Could you check a few things on this model? Use its own coordinates, in mm. Face numbers are marked on the shaded views. A direction names the side the tool comes from. Round coordinates to 2 decimals unless told otherwise and drop trailing zeros. Order: outer loops, then holes, each group sorted by start corner. A loop starts at its lowest first (then second) coordinate and runs counter-clockwise, first axis right, second up. Notation, with made-up numbers: M 26,84.25 L 40,84.25 A20 cw 40,110.25 Z; hole C 60,-14 d7. An arc over 180 degrees is marked long. Write each question's results on one line, items separated by ' | '. Start each with the question number.
1. Suppose I cut it at A-A on y = 176. Write out the boundary of the cut face in (x, z).
2. We'd pull the mould along X, two halves only. Please class the marked faces 1, 2 and 3: released by +X, released by -X, zero draft, split by the parting line, or undercut.
3. Suppose I cut it at B-B on x = 201. Write out the boundary of the cut face in (y, z), and give its area (3 significant figures).
4. I'm going to push a flat-ended pin straight in: pin 1 (1 mm diameter, centred on x = 204.5, y = 175.5, fed in from -Z). Where does the tip first touch, or does it pass through?
5. For the marked faces 4 and 5, which set-ups out of +Z, -Z, +X, -X, +Y, -Y let a thin tool reach every point of the face, with its end or its side?
6. Suppose I cut it at D-D on z = 1.4. Give the number of separate pieces and of enclosed holes in the cut face, and give its area (3 significant figures).
7. Please list where these lines run through material, in increasing order: L1, parallel to Y at x = 195, z = 0.85; L2, parallel to X at y = 164.5, z = 0.3; L3, parallel to X at y = 168.5, z = 2.
8. Suppose I cut it at C-C on y = 171. Write out the boundary of the cut face in (x, z), and give its area (3 significant figures).
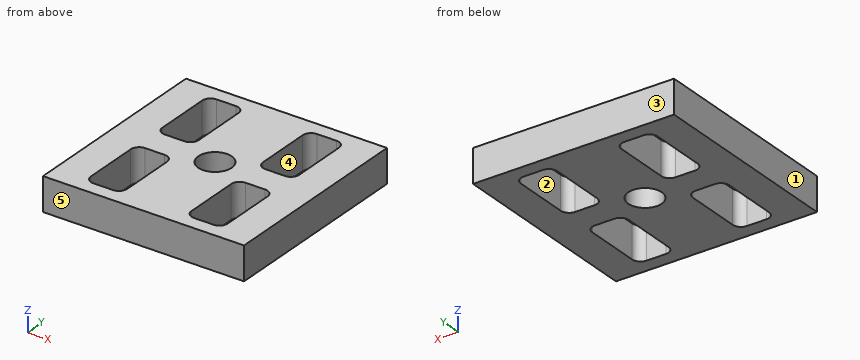
from build123d import *

# Parameters (mm, degrees)
MODEL_W                 = 18
MODEL_H                 = 18
MODEL_R                 = 1.5
SALIENTE_EXTRUIR1_DEPTH = 3


with BuildPart() as part:
    # Model → Saliente-Extruir1 (new body)
    with BuildSketch(Plane.XY):
        with Locations((199.835922194, 170.333196305)):
            Rectangle(MODEL_W, MODEL_H)
        with Locations((199.835922194, 170.333196305)):
            Circle(MODEL_R, mode=Mode.SUBTRACT)
        with BuildLine():
            Line((202.710922194, 172.333196305), (202.710922194, 177.333196305))
            ThreePointArc((202.710922194, 177.333196305), (202.930592108, 177.86352639), (203.460922194, 178.083196305))
            Line((203.460922194, 178.083196305), (205.210922194, 178.083196305))
            ThreePointArc((205.210922194, 178.083196305), (205.74125228, 177.86352639), (205.960922194, 177.333196305))
            Line((205.960922194, 177.333196305), (205.960922194, 172.333196305))
            ThreePointArc((205.960922194, 172.333196305), (205.74125228, 171.802866219), (205.210922194, 171.583196305))
            Line((205.210922194, 171.583196305), (203.460922194, 171.583196305))
            ThreePointArc((203.460922194, 171.583196305), (202.930592108, 171.802866219), (202.710922194, 172.333196305))
        make_face(mode=Mode.SUBTRACT)
        with BuildLine():
            Line((205.960922194, 168.333196305), (205.960922194, 163.333196305))
            ThreePointArc((205.960922194, 163.333196305), (205.74125228, 162.802866219), (205.210922194, 162.583196305))
            Line((205.210922194, 162.583196305), (203.460922194, 162.583196305))
            ThreePointArc((203.460922194, 162.583196305), (202.930592108, 162.802866219), (202.710922194, 163.333196305))
            Line((202.710922194, 163.333196305), (202.710922194, 168.333196305))
            ThreePointArc((202.710922194, 168.333196305), (202.930592108, 168.86352639), (203.460922194, 169.083196305))
            Line((203.460922194, 169.083196305), (205.210922194, 169.083196305))
            ThreePointArc((205.210922194, 169.083196305), (205.74125228, 168.86352639), (205.960922194, 168.333196305))
        make_face(mode=Mode.SUBTRACT)
        with BuildLine():
            Line((196.960922194, 168.333196305), (196.960922194, 163.333196305))
            ThreePointArc((196.960922194, 163.333196305), (196.74125228, 162.802866219), (196.210922194, 162.583196305))
            Line((196.210922194, 162.583196305), (194.460922194, 162.583196305))
            ThreePointArc((194.460922194, 162.583196305), (193.930592108, 162.802866219), (193.710922194, 163.333196305))
            Line((193.710922194, 163.333196305), (193.710922194, 168.333196305))
            ThreePointArc((193.710922194, 168.333196305), (193.930592108, 168.86352639), (194.460922194, 169.083196305))
            Line((194.460922194, 169.083196305), (196.210922194, 169.083196305))
            ThreePointArc((196.210922194, 169.083196305), (196.74125228, 168.86352639), (196.960922194, 168.333196305))
        make_face(mode=Mode.SUBTRACT)
        with BuildLine():
            Line((196.960922194, 177.333196305), (196.960922194, 172.333196305))
            ThreePointArc((196.960922194, 172.333196305), (196.74125228, 171.802866219), (196.210922194, 171.583196305))
            Line((196.210922194, 171.583196305), (194.460922194, 171.583196305))
            ThreePointArc((194.460922194, 171.583196305), (193.930592108, 171.802866219), (193.710922194, 172.333196305))
            Line((193.710922194, 172.333196305), (193.710922194, 177.333196305))
            ThreePointArc((193.710922194, 177.333196305), (193.930592108, 177.86352639), (194.460922194, 178.083196305))
            Line((194.460922194, 178.083196305), (196.210922194, 178.083196305))
            ThreePointArc((196.210922194, 178.083196305), (196.74125228, 177.86352639), (196.960922194, 177.333196305))
        make_face(mode=Mode.SUBTRACT)
    extrude(amount=SALIENTE_EXTRUIR1_DEPTH)


solid = part.part
Filled sheet:
1) outline: M 190.84,0 L 193.71,0 L 193.71,3 L 190.84,3 Z; M 196.96,0 L 202.71,0 L 202.71,3 L 196.96,3 Z; M 205.96,0 L 208.84,0 L 208.84,3 L 205.96,3 Z
2) face 1: released by -X | face 2: undercut | face 3: zero draft
3) outline: M 161.33,0 L 169.39,0 L 169.39,3 L 161.33,3 Z; M 171.28,0 L 179.33,0 L 179.33,3 L 171.28,3 Z | area: 48.3 mm^2
4) pin 1: passes through
5) face 4: +Z, -Z | face 5: +Z, -Z, +X, -X, -Y
6) separate pieces: 1 | enclosed holes: 5 | area: 234 mm^2
7) L1: y = 161.33 to 162.58, 169.08 to 171.58, 178.08 to 179.33 | L2: x = 190.84 to 193.71, 196.96 to 202.71, 205.96 to 208.84 | L3: x = 190.84 to 193.73, 196.94 to 202.73, 205.94 to 208.84
8) outline: M 190.84,0 L 198.49,0 L 198.49,3 L 190.84,3 Z; M 201.18,0 L 208.84,0 L 208.84,3 L 201.18,3 Z | area: 45.9 mm^2
